CAD build for the part. Positions are in the model's coordinates, mm. A direction names the side the tool comes from. Give positions to 0.01 mm unless a question says otherwise; leave off trailing zeros. Write each loop counter-clockwise with the first axis right and the second up, starting at its lowest first coordinate (ties: lowest second). Pieces come first, ordered by that corner, then holes. Notation, with made-up numbers: (81.5, 27.25) - (134.5, 27.25) arc R23 cw to (134.5, 63.25) - close; hole circle Ø3 at (-28.5, 2.25). An arc over 180 degrees is marked (long way). Answer as a JSON object with one key per item and string values.
from build123d import *

# Parameters (mm, degrees)
BOSS_EXTRUDE1_DEPTH     = 76.2
SKETCH3_R               = 1.397
CUT_EXTRUDE2_DEPTH      = 25.4
CUT_EXTRUDE4_REACH      = 81.348
CUT_EXTRUDE4_END_RADIUS = 94.615
SKETCH6_W               = 16.383
SKETCH6_H               = 25.4
SKETCH6_H_2             = 12.7
SKETCH7_R               = 1.397
CUT_EXTRUDE5_DEPTH      = 50.8


with BuildPart() as part:
    # Sketch1 → Boss-Extrude1 (new body)
    with BuildSketch(Plane(origin=(0, 0, 0), x_dir=(1, 0, 0), z_dir=(0, 1, 0))):
        with BuildLine():
            Line((-8.255, -94.254194602), (-8.255, -106.954194602))
            Line((-8.255, -106.954194602), (-1.905, -106.954194602))
            Line((-1.905, -106.954194602), (-1.905, -94.595820204))
            ThreePointArc((-1.905, -94.595820204), (-0.063512031, -94.614978683), (1.778, -94.598292485))
            Line((1.778, -94.598292485), (1.778, -106.954194602))
            Line((1.778, -106.954194602), (8.128, -106.954194602))
            Line((8.128, -106.954194602), (8.128, -94.265231348))
            ThreePointArc((8.128, -94.265231348), (10.397970458, -94.041907867), (12.661897921, -93.763929984))
            Line((12.661897921, -93.763929984), (11.398979566, -88.806415815))
            ThreePointArc((11.398979566, -88.806415815), (0, -89.535), (-11.398979566, -88.806415815))
            Line((-11.398979566, -88.806415815), (-12.661897921, -93.763929984))
            ThreePointArc((-12.661897921, -93.763929984), (-10.461321356, -94.034881722), (-8.255, -94.254194602))
        make_face()
    extrude(amount=BOSS_EXTRUDE1_DEPTH)

    # Sketch3 → Cut-Extrude2 (cut)
    with BuildSketch(Plane.ZY.offset(8.255)):
        with Locations((100.604194602, 57.15)):
            Circle(SKETCH3_R)
        with Locations((100.604194602, 19.05)):
            Circle(SKETCH3_R)
    extrude(amount=-CUT_EXTRUDE2_DEPTH, mode=Mode.SUBTRACT)

    # Cut-Extrude4: up to this cylinder (the profile starts outside it)
    cut_extrude4_end = Plane(origin=(0, 38.1, 0), z_dir=(0, -1, 0)) * Cylinder(CUT_EXTRUDE4_END_RADIUS, 416.426, mode=Mode.PRIVATE)
    # Sketch6 → Cut-Extrude4 (cut, up to the surface)
    with BuildSketch(Plane.XY.offset(106.954194602), mode=Mode.PRIVATE) as cut_extrude4_sk1:
        with Locations((-0.0635, 38.1)):
            Rectangle(SKETCH6_W, SKETCH6_H)
    cut_extrude4_tool1 = extrude(cut_extrude4_sk1.sketch, amount=-CUT_EXTRUDE4_REACH, mode=Mode.PRIVATE) - cut_extrude4_end
    add(cut_extrude4_tool1.solids().sort_by_distance((-0.0635, 38.1, 106.954195))[0], mode=Mode.SUBTRACT)
    # Sketch6 → Cut-Extrude4 (cut, up to the surface)
    with BuildSketch(Plane.XY.offset(106.954194602), mode=Mode.PRIVATE) as cut_extrude4_sk2:
        with Locations((-0.0635, 69.85)):
            Rectangle(SKETCH6_W, SKETCH6_H_2)
    cut_extrude4_tool2 = extrude(cut_extrude4_sk2.sketch, amount=-CUT_EXTRUDE4_REACH, mode=Mode.PRIVATE) - cut_extrude4_end
    add(cut_extrude4_tool2.solids().sort_by_distance((-0.0635, 69.85, 106.954195))[0], mode=Mode.SUBTRACT)
    # Sketch6 → Cut-Extrude4 (cut, up to the surface)
    with BuildSketch(Plane.XY.offset(106.954194602), mode=Mode.PRIVATE) as cut_extrude4_sk3:
        with Locations((-0.0635, 6.35)):
            Rectangle(SKETCH6_W, SKETCH6_H_2)
    cut_extrude4_tool3 = extrude(cut_extrude4_sk3.sketch, amount=-CUT_EXTRUDE4_REACH, mode=Mode.PRIVATE) - cut_extrude4_end
    add(cut_extrude4_tool3.solids().sort_by_distance((-0.0635, 6.35, 106.954195))[0], mode=Mode.SUBTRACT)

    # Sketch7 → Cut-Extrude5 (cut)
    with BuildSketch(Plane.XY.offset(106.954194602)):
        with Locations((0, 69.85)):
            Circle(SKETCH7_R)
        with Locations((0, 6.35)):
            Circle(SKETCH7_R)
    extrude(amount=-CUT_EXTRUDE5_DEPTH, mode=Mode.SUBTRACT)


solid = part.part
(1) Pull direction X, two halves, no side cores. Call faces 4 (the face through (8.128, 55.6, 100.7)), 5 (the face through (1.778, 55.6, 100.7)), 6 (the face through (-0.182, 7.735, 92.105)), 7 (the face through (5, 12.7, 101)): pulls with the +X half, pulls with the -X half, needs draft (parallel to the pull), parting line crosses it, or undercut.
Answer key:
{"face 4": "pulls with the +X half", "face 5": "undercut", "face 6": "undercut", "face 7": "needs draft"}
(2) Saw through at B-B, the plane x = 0. Give the cut face in (y, z) (3 decimals).
Answer key:
{"outline": "(0, 89.535) - (4.953, 89.535) - (4.953, 94.615) - (0, 94.615) - close; (7.747, 89.535) - (68.453, 89.535) - (68.453, 94.615) - (7.747, 94.615) - close; (71.247, 89.535) - (76.2, 89.535) - (76.2, 94.615) - (71.247, 94.615) - close"}
(3) Flat gauge pins, fed straight in: P1, Ø1.5, axis at x = 9.5, y = 46.5, coming from the +Z side; P2, Ø3.5, axis at y = 19.05, z = 100.6, coming from the +X side; P3, Ø5, axis at x = -6.5, y = 21.5, coming from the -Z side; P4, Ø2, axis at y = 57.15, z = 100.6, coming from the +X side. Where does each tip first touch, or does it go through?
Answer key:
{"P1": "stops at z = 94.21", "P2": "stops at x = 8.13", "P3": "stops at z = 89.08", "P4": "passes through"}
(4) Saw through at A-A, the plane y = 19.05. Give the cut face in (x, z) (3 decimals).
Answer key:
{"outline": "(-12.662, 93.764) - (-11.399, 88.806) arc R89.535 cw to (11.399, 88.806) - (12.662, 93.764) arc R94.615 ccw to (8.128, 94.265) - (8.128, 99.207) - (1.778, 99.207) - (1.778, 94.598) arc R94.615 ccw to (-1.905, 94.596) - (-1.905, 99.207) - (-8.255, 99.207) - (-8.255, 94.254) arc R94.615 ccw to start; (-8.255, 102.001) - (-1.905, 102.001) - (-1.905, 106.954) - (-8.255, 106.954) - close; (1.778, 102.001) - (8.128, 102.001) - (8.128, 106.954) - (1.778, 106.954) - close"}
(5) 3-axis set-ups, long thin cutter, end or side, ignore diameter. For faces 1 (the face through (-8.255, 55.6, 100.5)), 2 (the face through (1.778, 17.5, 100.7)), 3 (the face through (-12.02, 37.57, 91.25)): which of +Z, -Z, +X, -X, +Y, -Y reach the whole face in a straight line?
Answer key:
{"face 1": "+Z, -X, +Y, -Y", "face 2": "+Z, +Y, -Y", "face 3": "-Z, -X, +Y, -Y"}
(6) Probe L1, parallel to Y at x = 0, z = 92.4; L2, parallel to Y at x = 4.5, z = 103.75; L3, parallel to X at y = 56, z = 95.5 (3 decimals). List the from-to ranges inside material, lowest first. Write a range as [from, to].
Answer key:
{"L1": "y = [0, 4.95], [7.75, 68.45], [71.25, 76.2]", "L2": "y = [12.7, 25.4], [50.8, 63.5]", "L3": "x = [-8.255, -1.905], [1.778, 8.128]"}
(7) Saw through at C-C, the plane z = 97.25. Give the cut face in (x, y) (3 decimals).
Answer key:
{"outline": "(-8.255, 12.7) - (-1.905, 12.7) - (-1.905, 25.4) - (-8.255, 25.4) - close; (-8.255, 50.8) - (-1.905, 50.8) - (-1.905, 63.5) - (-8.255, 63.5) - close; (1.778, 12.7) - (8.128, 12.7) - (8.128, 25.4) - (1.778, 25.4) - close; (1.778, 50.8) - (8.128, 50.8) - (8.128, 63.5) - (1.778, 63.5) - close"}
(8) Saw through at D-D, the plane x = -5.5. Give the cut face in (y, z) (3 decimals).
Answer key:
{"outline": "(0, 89.366) - (76.2, 89.366) - (76.2, 94.455) - (63.5, 94.455) - (63.5, 106.954) - (50.8, 106.954) - (50.8, 94.455) - (25.4, 94.455) - (25.4, 106.954) - (12.7, 106.954) - (12.7, 94.455) - (0, 94.455) - close; hole circle Ø2.794 at (19.05, 100.604); hole circle Ø2.794 at (57.15, 100.604)"}
